from build123d import *

# Parameters (mm, degrees)
SKETCH1_W           = 28
SKETCH1_H           = 27
BOSS_EXTRUDE1_DEPTH = 45
SKETCH2_W           = 22.4
SKETCH2_H           = 21.6
CUT_EXTRUDE1_DEPTH  = 43
FILLET3_R           = 2
SKETCH12_W          = 28
SKETCH12_H          = 3.238807787
CUT_EXTRUDE9_DEPTH  = 50.022953807


with BuildPart() as part:
    # Sketch1 → Boss-Extrude1 (new body)
    with BuildSketch(Plane.XY):
        Rectangle(SKETCH1_W, SKETCH1_H)
    extrude(amount=BOSS_EXTRUDE1_DEPTH)

    # Sketch2 → Cut-Extrude1 (cut)
    with BuildSketch(Plane.XY.offset(45)):
        Rectangle(SKETCH2_W, SKETCH2_H)
    extrude(amount=-CUT_EXTRUDE1_DEPTH, mode=Mode.SUBTRACT)

    # Fillet3
    fillet3_edges = [part.edges().sort_by_distance(p)[0] for p in [
        (-14, 13.5, 22.5),
        (14, 13.5, 22.5),
    ]]
    fillet(fillet3_edges, radius=FILLET3_R)

    # Sketch12 → Cut-Extrude9 (cut, through all)
    with BuildSketch(Plane.XY.offset(45)):
        with Locations((0, 12.419403894)):
            Rectangle(SKETCH12_W, SKETCH12_H)
    extrude(amount=-CUT_EXTRUDE9_DEPTH, mode=Mode.SUBTRACT)


solid = part.part
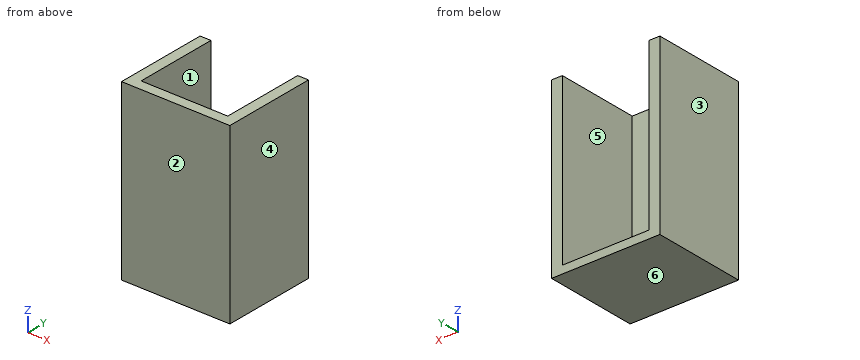
Part model, mm, in its own coordinate system. Face numbers are marked on the shaded views. A direction names the side the tool comes from. Give positions to 0.01 mm unless a question says otherwise; leave off trailing zeros. Loops run counter-clockwise (first coordinate to the right, second up) from the corner with the lowest first, then second, coordinate; pieces in that order, holes last. Notation, with made-up numbers: M -10,15 L 20,15 A16 ccw 20,24 Z; hole C -14,-16.75 d6. An arc over 180 degrees is marked long. Put each result on its own line as item: value. Start each with the question number.
1) Saw through at C-C (x = 3.5). List the corners of the cut face in (y, z).
2) Pull direction X, two halves, no side cores. Call the marked faces 1, 2, 3 and 4: +X half, -X half, draft (parallel to the pull), parting line (faces both ways), or undercut.
3) Flat gauge pins, fed straight in: pin 1 (1 mm diameter, centred on x = 1.5, y = 0.5, fed in from -Z); pin 2 (3 mm diameter, centred on x = -4.5, z = 25.5, fed in from +Y). Where does each tip first touch, or does it go through?
4) Probe probe 1 along X at (y, z) = (5.5, 16.5); probe 2 along Z at (x, y) = (-8, 1); probe 3 along Y at (x, z) = (-9, 14). List the from-to ranges inside material, lowest first.
5) Saw through at B-B (z = 41). List the corners of the cut face in (x, y).
6) 3-axis set-ups, long thin cutter, end or side, ignore diameter. For the marked faces 5 and 6: which of +Z, -Z, +X, -X, +Y, -Y reach the whole face in a straight line?
7) Saw through at A-A (y = 9). List the corners of the cut face in (x, z).
Numbers:
1. outline: M -13.5,0 L 10.8,0 L 10.8,2 L -10.8,2 L -10.8,45 L -13.5,45 Z
2. face 1: undercut
2. face 2: draft
2. face 3: -X half
2. face 4: +X half
3. pin 1: z = 0
3. pin 2: y = -10.8
4. probe 1: -14 to -11.2, 11.2 to 14
4. probe 2: 0 to 2
4. probe 3: -13.5 to -10.8
5. outline: M -14,-13.5 L 14,-13.5 L 14,10.8 L 11.2,10.8 L 11.2,-10.8 L -11.2,-10.8 L -11.2,10.8 L -14,10.8 Z
6. face 5: +Z, +Y
6. face 6: -Z, +X, -X, +Y, -Y
7. outline: M -14,0 L 14,0 L 14,45 L 11.2,45 L 11.2,2 L -11.2,2 L -11.2,45 L -14,45 Z
